For this review, use the dimensioned drawing (mm, ordinates from the lowest corner) and the shaded views. A direction names the side the tool comes from. Coordinates: 2 decimals unless noted, no trailing zeros. Loops run counter-clockwise (first coordinate to the right, second up) from the corner with the lowest first, then second, coordinate; pieces in that order, holes last. Notation, with made-up numbers: M -6.5,5 L 32.5,5 A19 ccw 32.5,38 Z; hole C 85.5,4 d3. An arc over 180 degrees is marked long. One line per item, written item: value.
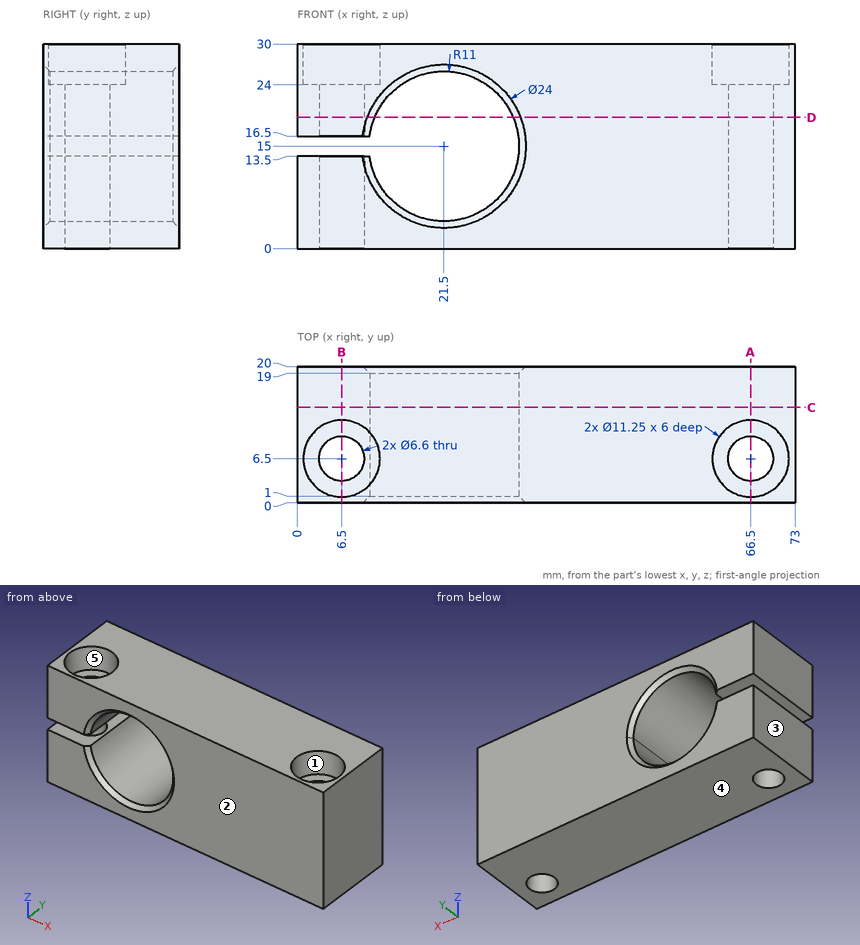
(1) Mouldability with a two-part tool opening along X and no side actions: class the marked faces 1, 2 and 3 as released by +X, released by -X, zero draft, split by the parting line, or undercut.
Reply:
face 1: undercut
face 2: zero draft
face 3: released by -X
(2) Tool access review of the marked faces 4 and 5: name each direction out of +Z, -Z, +X, -X, +Y, -Y from which nothing blocks a thin tool from reaching the whole face with its end or side.
Reply:
face 4: -Z, +X, -X, +Y, -Y
face 5: +Z
(3) We need section A-A on x = 66.5. State the section outline as (y, z) points (3 decimals).
Reply:
outline: M 0,0 L 3.2,0 L 3.2,24 L 0.875,24 L 0.875,30 L 0,30 Z; M 9.8,0 L 20,0 L 20,30 L 12.125,30 L 12.125,24 L 9.8,24 Z
(4) Insertion check: pin 1 (7.5 mm diameter, centred on x = 66.5, y = 6.5, fed in from +Z). The pin has a flat end and moves straight along its axis. Give the tip position at first contact, or say it passes through.
Reply:
pin 1: stops at z = 24
(5) We need section B-B on x = 6.5. State the section outline as (y, z) points (3 decimals).
Reply:
outline: M 0,0 L 3.2,0 L 3.2,13.5 L 0,13.5 Z; M 0,16.5 L 3.2,16.5 L 3.2,24 L 0.875,24 L 0.875,30 L 0,30 Z; M 9.8,0 L 20,0 L 20,13.5 L 9.8,13.5 Z; M 9.8,16.5 L 20,16.5 L 20,30 L 12.125,30 L 12.125,24 L 9.8,24 Z
(6) We need section C-C on y = 14. State the section outline as (x, z) points.
Reply:
outline: M 0,0 L 73,0 L 73,30 L 0,30 L 0,16.5 L 10.6,16.5 A11 cw long 10.6,13.5 L 0,13.5 Z
(7) To check wall thickness, follow line 1 along Y through (x, z) = (6.5, 4.5); line 2 along Z through (x, y) = (5, 1.25); line 3 along Y through (x, z) = (6.5, 25.3) (3 decimals). State the ranges of each line that lie inside material, in increasing order. Write a range as [from, to].
Reply:
line 1: y = [0, 3.2], [9.8, 20]
line 2: z = [0, 13.5], [16.5, 24]
line 3: y = [0, 0.875], [12.125, 20]
(8) We need section D-D on z = 19.25. State how many separate pieces and enclosed holes the cut face has, then the cut area to 3 significant figures.
Reply:
separate pieces: 2
enclosed holes: 2
area: 984 mm2
